The drawing under review shows one solid part. Ordinate dimensions are in mm from its lowest x, y, z. A direction names the side the tool comes from. Give positions to 0.01 mm unless a question says otherwise; leave off trailing zeros. Order: outer loops, then holes, each group sorted by start corner. A loop starts at its lowest first (then second) coordinate and runs counter-clockwise, first axis right, second up. Notation, with made-up numbers: (28, -39.75) -> (54, -39.75) arc R16 cw to (54, -23.75) -> close; hole circle Ø7 at (-12, 78.25). An arc over 180 degrees is marked (long way). One line per item, written item: value. Start each with the question number.
1) Consider section A-A (x = 12). State the section outline as (y, z) points.
2) Consider section C-C (z = 2.3). State the section outline as (x, y) points, plus the area to 3 significant figures.
3) Wall thickness on line 1 along Y through (x, z) = (12, 2.2); line 2 along Y through (x, z) = (4.25, 2.4); line 3 along X through (y, z) = (0.5, 1.5) (1 decimal): over which ranges is each line inside the solid? List them lowest first. Write a range as from..to.
4) The part is to be moulded in two halves that separate along Y. For the marked faces 3, 4 and 5, say which applies: released by +Y, released by -Y, zero draft, split by the parting line, or undercut.
5) For pin 1 (1.8 mm diameter, centred on x = 12, y = 6, fed in from -Z); pin 2 (1.5 mm diameter, centred on x = 4.5, z = 2, fed in from +Y), all flat-tipped, find the tip position at first contact; note any pin that passes through.
6) Tool access review of the marked faces 1 and 2: name each direction out of +Z, -Z, +X, -X, +Y, -Y from which nothing blocks a thin tool from reaching the whole face with its end or side.
7) Consider section B-B (y = 6). State the section outline as (x, z) points.
8) Consider section D-D (x = 4.75). State the section outline as (y, z) points, plus the area to 3 significant figures.
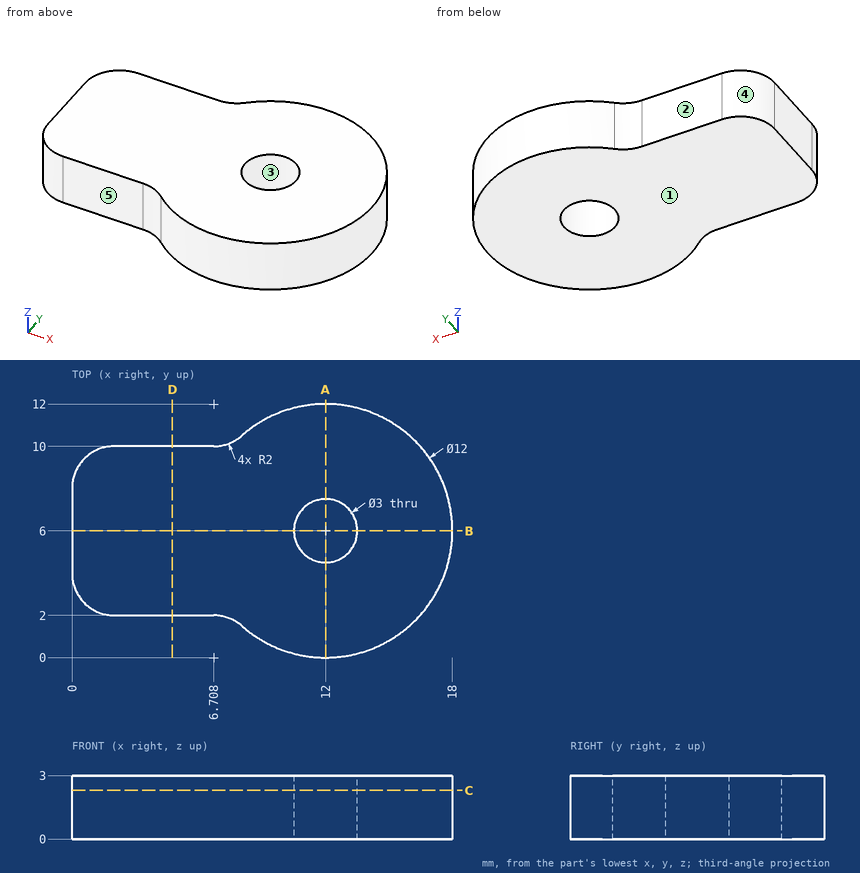
Checked values:
1. outline: (0, 0) -> (4.5, 0) -> (4.5, 3) -> (0, 3) -> close; (7.5, 0) -> (12, 0) -> (12, 3) -> (7.5, 3) -> close
2. outline: (0, 4) arc R2 ccw to (2, 2) -> (6.71, 2) arc R2 cw to (8.03, 1.5) arc R6 ccw (long way) to (8.03, 10.5) arc R2 cw to (6.71, 10) -> (2, 10) arc R2 ccw to (0, 8) -> close; hole circle Ø3 at (12, 6)
2. area: 156 mm^2
3. line 1: y = 0..4.5, 7.5..12
3. line 2: y = 2..10
3. line 3: x = 9.6..14.4
4. face 3: undercut
4. face 4: released by +Y
4. face 5: released by -Y
5. pin 1: passes through
5. pin 2: stops at y = 10
6. face 1: -Z, +X, -X, +Y, -Y
6. face 2: +Z, -Z, -X, +Y
7. outline: (0, 0) -> (10.5, 0) -> (10.5, 3) -> (0, 3) -> close; (13.5, 0) -> (18, 0) -> (18, 3) -> (13.5, 3) -> close
8. outline: (2, 0) -> (10, 0) -> (10, 3) -> (2, 3) -> close
8. area: 24.0 mm^2
